CAD build for the part. Positions are in the model's coordinates, mm. Face numbers are marked on the shaded views. Round coordinates to 2 decimals unless told otherwise and drop trailing zeros. Order: outer loops, then holes, each group sorted by start corner. A loop starts at its lowest first (then second) coordinate and runs counter-clockwise, first axis right, second up. Notation, with made-up numbers: M 57.25,7.25 L 116.25,7.25 A26 ccw 116.25,23.25 Z; hole C 38,85 d7. An arc over 180 degrees is marked long. Answer as a JSON object with one key per item and string values. Group by question number.
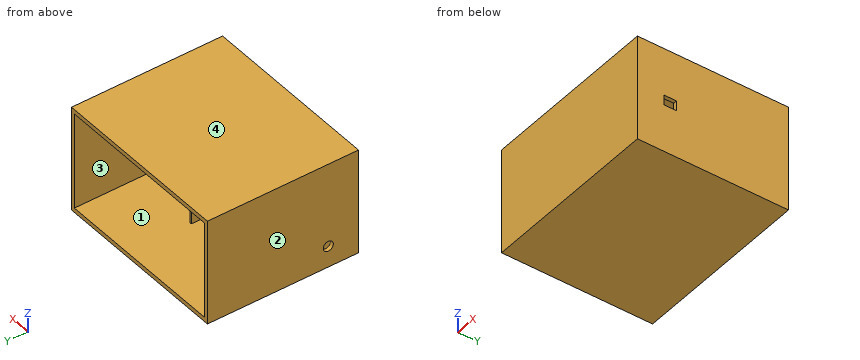
```python
from build123d import *

# Parameters (mm, degrees)
SKETCH1_W           = 144
SKETCH1_H           = 84
BOSS_EXTRUDE1_DEPTH = 120
SKETCH2_W           = 138
SKETCH2_H           = 77
CUT_EXTRUDE1_DEPTH  = 100
SKETCH3_R           = 4
CUT_EXTRUDE3_DEPTH  = 50
SKETCH5_W           = 8
SKETCH5_H           = 10
CUT_EXTRUDE4_DEPTH  = 20
SKETCH4_W           = 32
SKETCH4_H           = 12
BOSS_EXTRUDE4_DEPTH = 45
SKETCH4_2_W         = 32
SKETCH4_2_H         = 12
BOSS_EXTRUDE5_DEPTH = 45
SKETCH11_W          = 29
SKETCH11_H          = 10
CUT_EXTRUDE5_DEPTH  = 45


with BuildPart() as part:
    # Sketch1 → Boss-Extrude1 (new body)
    with BuildSketch(Plane(origin=(0, 0, 0), x_dir=(1, 0, 0), z_dir=(0, 1, 0))):
        Rectangle(SKETCH1_W, SKETCH1_H)
    extrude(amount=BOSS_EXTRUDE1_DEPTH)

    # Sketch2 → Cut-Extrude1 (cut)
    with BuildSketch(Plane(origin=(0, 120, 0), x_dir=(1, 0, 0), z_dir=(0, 1, 0))):
        Rectangle(SKETCH2_W, SKETCH2_H)
    extrude(amount=-CUT_EXTRUDE1_DEPTH, mode=Mode.SUBTRACT)

    # Sketch3 → Cut-Extrude3 (cut, symmetric)
    with BuildSketch(Plane.ZY.offset(72)):
        with Locations(Location((-25, 24, 0), (0, 0, 270))):
            Circle(SKETCH3_R)
    extrude(amount=CUT_EXTRUDE3_DEPTH, both=True, mode=Mode.SUBTRACT)

    # Sketch5 → Cut-Extrude4 (cut, symmetric)
    with BuildSketch(Plane(origin=(72, 0, 0), x_dir=(0, 0, -1), z_dir=(1, 0, 0))):
        with Locations((0, 26)):
            Rectangle(SKETCH5_W, SKETCH5_H)
    extrude(amount=CUT_EXTRUDE4_DEPTH, both=True, mode=Mode.SUBTRACT)

    # Sketch4 → Boss-Extrude4 (add)
    with BuildSketch(Plane(origin=(0, 25, 0), x_dir=(1, 0, 0), z_dir=(0, 1, 0))):
        with Locations((-3, 32.5)):
            Rectangle(SKETCH4_W, SKETCH4_H)
    extrude(amount=BOSS_EXTRUDE4_DEPTH)

    # Sketch4_2 → Boss-Extrude5 (add)
    with BuildSketch(Plane(origin=(0, 25, 0), x_dir=(1, 0, 0), z_dir=(0, 1, 0))):
        with Locations((-3, 32.5)):
            Rectangle(SKETCH4_2_W, SKETCH4_2_H)
    extrude(amount=BOSS_EXTRUDE5_DEPTH)

    # Sketch11 → Cut-Extrude5 (cut)
    with BuildSketch(Plane(origin=(0, 70, 0), x_dir=(1, 0, 0), z_dir=(0, 1, 0))):
        with Locations((-2.873413599, 33.5)):
            Rectangle(SKETCH11_W, SKETCH11_H)
    extrude(amount=-CUT_EXTRUDE5_DEPTH, mode=Mode.SUBTRACT)


solid = part.part
```
Item 1: Cut at D-D, the plane y = 98.5. Give the cut face in (x, z), and give its area (3 significant figures).
Item 2: Cut at A-A, the plane x = -60. Give the cut face in (y, z), and give its area (3 significant figures).
Item 3: Two-plate mould, pull along X, no slides. Class the marked faces 1, 2, 3 and 4: +X half, -X half, draft (parallel to the pull), parting line (faces both ways), or undercut.
Item 4: Flat gauge pin, fed straight in: pin 1 Ø2 at (x, z) = (20, -24) entering from +Y. Where does the tip first touch, or does it go through?
Item 5: Cut at B-B, the plane z = 1.5. Give the cut face in (x, y).
Item 6: Drill centre lines: line 1 (X direction, y = 42.5, z = -33); line 2 (X direction, y = 42, z = 20); line 3 (Z direction, x = 58.5, y = 89.5). Where is each one in solid material? Low to high. Write a range as [from, to].
Item 7: Cut at C-C, the plane y = 45. Give the cut face in (x, z).
Response values:
{
 "1": {"outline": "M -72,-42 L 72,-42 L 72,42 L -72,42 Z; hole M -69,-38.5 L 69,-38.5 L 69,38.5 L -69,38.5 Z", "area": "1,470 mm^2"},
 "2": {"outline": "M 0,-42 L 120,-42 L 120,-38.5 L 20,-38.5 L 20,38.5 L 120,38.5 L 120,42 L 0,42 Z", "area": "2,380 mm^2"},
 "3": {"face 1": "undercut", "face 2": "-X half", "face 3": "undercut", "face 4": "draft"},
 "4": {"pin 1": "y = 20"},
 "5": {"outline": "M -72,0 L 72,0 L 72,21 L 69,21 L 69,20 L -69,20 L -69,120 L -72,120 Z; M 69,31 L 72,31 L 72,120 L 69,120 Z"},
 "6": {"line 1": "[-72, -69], [-19, -17.37], [11.63, 13], [69, 72]", "line 2": "[-72, -69], [69, 72]", "line 3": "[-42, -38.5], [38.5, 42]"},
 "7": {"outline": "M -72,-42 L 72,-42 L 72,42 L -72,42 Z; hole M -69,-38.5 L -19,-38.5 L -19,-26.5 L 13,-26.5 L 13,-38.5 L 69,-38.5 L 69,38.5 L -69,38.5 Z; hole M -17.37,-38.5 L 11.63,-38.5 L 11.63,-28.5 L -17.37,-28.5 Z"}
}
